Geometry: final body of the model. Coordinates: model frame, mm. A direction names the side the tool comes from. Give positions to 0.01 mm unless a question says otherwise; leave off trailing zeros. One line per item, written item: value.
```python
from build123d import *
from build123d.topology import SkipClean

# Parameters (mm, degrees)
SKETCH_1_W          = 130
SKETCH_1_H          = 180
SKETCH_1_R          = 1.65
SKETCH_1_R_2        = 4.9
SKETCH_1_R_3        = 2.625
SKETCH_1_R_4        = 15
SKETCH_1_W_2        = 80
SKETCH_1_H_2        = 4
EXTRUDE_1_DEPTH     = 3
SKETCH_3_R          = 1.65
CUT_EXTRUDE_2_DEPTH = 112.05854312
SKETCH_4_W          = 15
SKETCH_4_H          = 10.5
CUT_EXTRUDE_3_DEPTH = 2.51
SKETCH_5_W          = 14.05
SKETCH_5_H          = 8.1
CUT_EXTRUDE_4_DEPTH = 0.49
EXTRUDE_START       = 45
SKETCH_6_W          = 25
SKETCH_6_H          = 1
EXTRUDE_2_DEPTH     = 40
SKETCH_9_R          = 2.625
CUT_EXTRUDE_5_DEPTH = 1
EXTRUDE_START_2     = -3
EXTRUDE_3_DEPTH     = 10
SKETCH_11_R         = 1.65
CUT_EXTRUDE_6_DEPTH = 133
SKETCH_12_R         = 3.1
CUT_EXTRUDE_7_DEPTH = 0.5
SKETCH_13_W         = 80
SKETCH_13_H         = 8
CUT_EXTRUDE_8_DEPTH = 3


with BuildPart() as part:
    # 草图1 → 凸台-拉伸1 (new body)
    with BuildSketch(Plane(origin=(0, 0, 0), x_dir=(1, 0, 0), z_dir=(0, 1, 0))):
        Rectangle(SKETCH_1_W, SKETCH_1_H)
        with Locations(Location((41.15, 34.063716669, 0), (0, 0, 90))):
            Circle(SKETCH_1_R, mode=Mode.SUBTRACT)
        with Locations(Location((55.15, 34.063716669, 0), (0, 0, 90))):
            Circle(SKETCH_1_R, mode=Mode.SUBTRACT)
        with Locations(Location((48.2, 42.063716669, 0), (0, 0, 90))):
            Circle(SKETCH_1_R_2, mode=Mode.SUBTRACT)
        with Locations(Location((41.15, 50.063716669, 0), (0, 0, 90))):
            Circle(SKETCH_1_R, mode=Mode.SUBTRACT)
        with Locations(Location((55.15, 50.063716669, 0), (0, 0, 90))):
            Circle(SKETCH_1_R, mode=Mode.SUBTRACT)
        with Locations(Location((-18, -51, 0), (0, 0, 270))):
            Circle(SKETCH_1_R_3, mode=Mode.SUBTRACT)
        with Locations(Location((18, -51, 0), (0, 0, 270))):
            Circle(SKETCH_1_R_3, mode=Mode.SUBTRACT)
        with Locations(Location((18, -79, 0), (0, 0, 270))):
            Circle(SKETCH_1_R_3, mode=Mode.SUBTRACT)
        with Locations(Location((-18, -79, 0), (0, 0, 270))):
            Circle(SKETCH_1_R_3, mode=Mode.SUBTRACT)
        with Locations(Location((0, -65, 0), (0, 0, 270))):
            Circle(SKETCH_1_R_4, mode=Mode.SUBTRACT)
        with Locations(Location((-41.15, 34.063716669, 0), (0, 0, 270))):
            Circle(SKETCH_1_R, mode=Mode.SUBTRACT)
        with Locations(Location((-55.15, 34.063716669, 0), (0, 0, 270))):
            Circle(SKETCH_1_R, mode=Mode.SUBTRACT)
        with Locations(Location((-55.15, 50.063716669, 0), (0, 0, 270))):
            Circle(SKETCH_1_R, mode=Mode.SUBTRACT)
        with Locations(Location((-48.2, 42.063716669, 0), (0, 0, 270))):
            Circle(SKETCH_1_R_2, mode=Mode.SUBTRACT)
        with Locations(Location((-41.15, 50.063716669, 0), (0, 0, 270))):
            Circle(SKETCH_1_R, mode=Mode.SUBTRACT)
        with Locations((0, -15.5)):
            Rectangle(SKETCH_1_W_2, SKETCH_1_H_2, mode=Mode.SUBTRACT)
        with Locations((0, 17.5)):
            Rectangle(SKETCH_1_W_2, SKETCH_1_H_2, mode=Mode.SUBTRACT)
    extrude(amount=EXTRUDE_1_DEPTH)

    # 草图3 → 切除-拉伸2 (cut, through all)
    with BuildSketch(Plane(origin=(0, 0, 0), x_dir=(1, 0, 0), z_dir=(0, 1, 0))):
        with Locations(Location((-34, 64, 0), (0, 0, 270))):
            Circle(SKETCH_3_R)
        with Locations(Location((-34, -4, 0), (0, 0, 270))):
            Circle(SKETCH_3_R)
        with Locations(Location((34, -4, 0), (0, 0, 90))):
            Circle(SKETCH_3_R)
        with Locations(Location((34, 64, 0), (0, 0, 90))):
            Circle(SKETCH_3_R)
        with Locations(Location((-51, -25, 0), (0, 0, 270))):
            Circle(SKETCH_3_R)
        with Locations(Location((-51.004420949, -69.2, 0), (0, 0, 270))):
            Circle(SKETCH_3_R)
        with Locations(Location((51.004420949, -69.2, 0), (0, 0, 90))):
            Circle(SKETCH_3_R)
        with Locations(Location((51, -25, 0), (0, 0, 90))):
            Circle(SKETCH_3_R)
    extrude(amount=CUT_EXTRUDE_2_DEPTH, mode=Mode.SUBTRACT)

    # 草图4 → 切除-拉伸3 (cut)
    with BuildSketch(Plane.XZ):
        with Locations((0, -80.75)):
            Rectangle(SKETCH_4_W, SKETCH_4_H)
    extrude(amount=-CUT_EXTRUDE_3_DEPTH, mode=Mode.SUBTRACT)

    # 草图5 → 切除-拉伸4 (cut)
    with BuildSketch(Plane.XZ.offset(-2.51)):
        with Locations((0, -80.75)):
            Rectangle(SKETCH_5_W, SKETCH_5_H)
    extrude(amount=-CUT_EXTRUDE_4_DEPTH, mode=Mode.SUBTRACT)

    # 草图6 → 凸台-拉伸2 (add)
    with BuildSketch(Plane.XY.offset(EXTRUDE_START)):
        with Locations((-12.5, -0.5)):
            Rectangle(SKETCH_6_W, SKETCH_6_H)
        with Locations((12.5, -0.5)):
            Rectangle(SKETCH_6_W, SKETCH_6_H)
    extrude(amount=EXTRUDE_2_DEPTH)

    # 草图9 → 切除-拉伸5 (cut)
    with SkipClean():  # the faces are left unmerged after this step: merging them gives an invalid solid
        with BuildSketch(Plane.XZ.offset(1)):
            with Locations(Location((-18, 51, 0), (0, 0, 270))):
                Circle(SKETCH_9_R)
            with Locations(Location((18, 51, 0), (0, 0, 270))):
                Circle(SKETCH_9_R)
            with Locations(Location((-18, 79, 0), (0, 0, 270))):
                Circle(SKETCH_9_R)
            with Locations(Location((18, 79, 0), (0, 0, 270))):
                Circle(SKETCH_9_R)
        extrude(amount=-CUT_EXTRUDE_5_DEPTH, mode=Mode.SUBTRACT)

    # 草图10 → 凸台-拉伸3 (add)
    with SkipClean():  # the faces are left unmerged after this step: merging them gives an invalid solid
        with BuildSketch(Plane(origin=(0, 3, 0), x_dir=(1, 0, 0), z_dir=(0, 1, 0)).offset(EXTRUDE_START_2)):
            with BuildLine():
                Line((-65, 63), (-67, 63))
                ThreePointArc((-67, 63), (-67.707106781, 62.707106781), (-68, 62))
                Line((-68, 62), (-68, -89))
                ThreePointArc((-68, -89), (-67.707106781, -89.707106781), (-67, -90))
                Line((-67, -90), (-65, -90))
                Line((-65, -90), (-65, 63))
            make_face()
            with BuildLine():
                Line((65, -90), (65, 63))
                Line((65, 63), (67, 63))
                ThreePointArc((67, 63), (67.707106781, 62.707106781), (68, 62))
                Line((68, 62), (68, -89))
                ThreePointArc((68, -89), (67.707106781, -89.707106781), (67, -90))
                Line((67, -90), (65, -90))
            make_face()
        extrude(amount=EXTRUDE_3_DEPTH)

    # 草图11 → 切除-拉伸6 (cut)
    with SkipClean():  # the faces are left unmerged after this step: merging them gives an invalid solid
        with BuildSketch(Plane(origin=(68, 0, 0), x_dir=(0, 0, -1), z_dir=(1, 0, 0))):
            with Locations((-33.5, 6)):
                Circle(SKETCH_11_R)
            with Locations((-68, 6)):
                Circle(SKETCH_11_R)
            with Locations((6.5, 6)):
                Circle(SKETCH_11_R)
            with Locations((41, 6)):
                Circle(SKETCH_11_R)
        cut_extrude_6 = extrude(amount=-CUT_EXTRUDE_6_DEPTH, mode=Mode.SUBTRACT)

    # 镜向1: 切除-拉伸6 across plane
    with SkipClean():  # the faces are left unmerged after this step: merging them gives an invalid solid
        add(cut_extrude_6.mirror(Plane(origin=(0, 0, 0), x_dir=(0, 0, 1), z_dir=(1, 0, 0))), mode=Mode.SUBTRACT)

    # 草图12 → 切除-拉伸7 (cut)
    with SkipClean():  # the faces are left unmerged after this step: merging them gives an invalid solid
        with BuildSketch(Plane(origin=(68, 0, 0), x_dir=(0, 0, -1), z_dir=(1, 0, 0))):
            with Locations((-68, 6)):
                Circle(SKETCH_12_R)
            with Locations((-33.5, 6)):
                Circle(SKETCH_12_R)
            with Locations((6.5, 6)):
                Circle(SKETCH_12_R)
            with Locations((41, 6)):
                Circle(SKETCH_12_R)
        cut_extrude_7 = extrude(amount=-CUT_EXTRUDE_7_DEPTH, mode=Mode.SUBTRACT)

    # 镜向3: 切除-拉伸7 across plane
    with SkipClean():  # the faces are left unmerged after this step: merging them gives an invalid solid
        add(cut_extrude_7.mirror(Plane(origin=(0, 0, 0), x_dir=(0, 0, 1), z_dir=(1, 0, 0))), mode=Mode.SUBTRACT)

    # 草图13 → 切除-拉伸8 (cut)
    with SkipClean():  # the faces are left unmerged after this step: merging them gives an invalid solid
        with BuildSketch(Plane(origin=(0, 3, 0), x_dir=(1, 0, 0), z_dir=(0, 1, 0))):
            with Locations((0, -15.5)):
                Rectangle(SKETCH_13_W, SKETCH_13_H)
            with Locations((0, 17.5)):
                Rectangle(SKETCH_13_W, SKETCH_13_H)
        extrude(amount=-CUT_EXTRUDE_8_DEPTH, mode=Mode.SUBTRACT)


solid = part.part
```
1) First-contact query: pin 1 (5.5 mm diameter, centred on x = 41.15, z = -50.06, fed in from -Y); pin 2 (5 mm diameter, centred on y = 4.5, z = -41, fed in from +X); pin 3 (9 mm diameter, centred on x = 2, z = 70, fed in from +Y); pin 4 (3.5 mm diameter, centred on y = 1, z = -71.5, fed in from +X). Flat tips, straight axial feed; report the tip coordinate or a pass-through.
Answers below:
pin 1: y = 0
pin 2: x = 68
pin 3: y = 0
pin 4: x = 65
2) Set-up query: faces 4 (the face through (67.754, 4.813, -43.864)), 5 (the face through (-1, 2.51, -85)), 6 (the face through (-67.5, 5, 32)). Return all of +Z, -Z, +X, -X, +Y, -Y with unobstructed straight access to the full face (end or side cutting, diameter ignored); none if empty.
Answers below:
face 4: +X
face 5: -Y
face 6: -X
3) Mould query, pull axis X, two halves, no side actions, for faces 1 (the face through (-46.7, 1.5, -37.4)), 2 (the face through (67.5, 5, -8)), 3 (the face through (-67.754, 4.114, 35.96)). Classes: released by +X, released by -X, zero draft, split by the parting line, or undercut.
Answers below:
face 1: undercut
face 2: released by +X
face 3: zero draft
4) Material intervals for line 1 along X through (y, z) = (-0.7, 51) (3 decimals); line 2 along Z through (x, y) = (-18, -0.45) (3 decimals); line 3 along X through (y, z) = (7.25, -45), sorted ascending.
Answers below:
line 1: -25 to -20.625, -15.375 to 15.375, 20.625 to 25
line 2: 45 to 48.375, 53.625 to 76.375, 81.625 to 85
line 3: -68 to -65, 65 to 68
